Answer from the drawing. Dimensions are ordinates in mm from the lowest x, y and z of the part. A direction names the side the tool comes from. Round coordinates to 2 decimals unless told otherwise and drop trailing zeros. Loops run counter-clockwise (first coordinate to the right, second up) from the corner with the lowest first, then second, coordinate; pieces in that order, holes last.
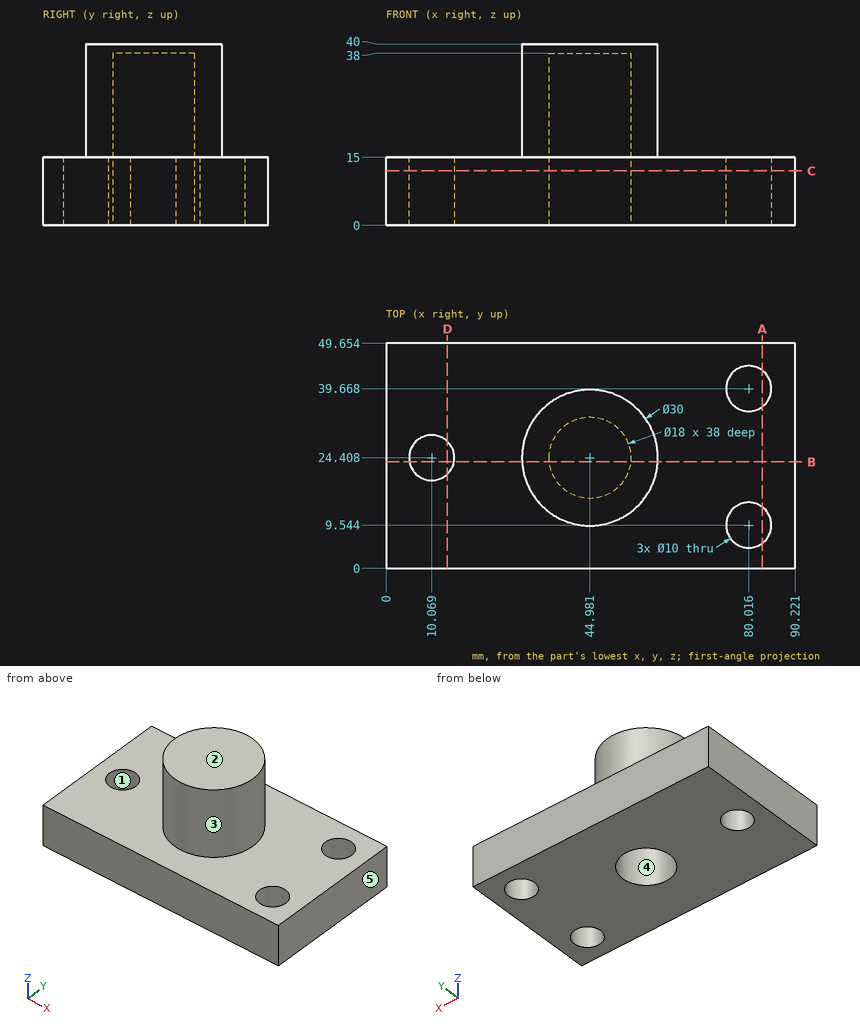
1. Find section B-B (y = 23.5). Write down the section's boundary in (x, z) (1 decimal).
Answer key:
outline: (0, 0) - (5.2, 0) - (5.2, 15) - (0, 15) - close; (15, 0) - (36, 0) - (36, 38) - (53.9, 38) - (53.9, 0) - (90.2, 0) - (90.2, 15) - (60, 15) - (60, 40) - (30, 40) - (30, 15) - (15, 15) - close
2. Find section A-A (x = 83). Write down the section's boundary in (y, z) (1 decimal).
Answer key:
outline: (0, 0) - (5.5, 0) - (5.5, 15) - (0, 15) - close; (13.6, 0) - (35.7, 0) - (35.7, 15) - (13.6, 15) - close; (43.7, 0) - (49.7, 0) - (49.7, 15) - (43.7, 15) - close
3. Find section C-C (z = 12). Write down the section's boundary in (x, y) (1 decimal).
Answer key:
outline: (0, 0) - (90.2, 0) - (90.2, 49.7) - (0, 49.7) - close; hole circle Ø10 at (10.1, 24.4); hole circle Ø18 at (45, 24.4); hole circle Ø10 at (80, 9.5); hole circle Ø10 at (80, 39.7)
4. Consider probe 1 along Z at (x, y) = (58.5, 3.5); probe 2 along X at (y, z) = (40, 8.5) (1 decimal); probe 3 along Y at (x, z) = (43, 6) (1 decimal). Determine where each line is inside the solid, lowest interval first.
Answer key:
probe 1: z = 0 to 15
probe 2: x = 0 to 75, 85 to 90.2
probe 3: y = 0 to 15.6, 33.2 to 49.7
5. Given pin 1 (4 mm diameter, centred on y = 27, z = 33, fed in from +X); pin 2 (6 mm diameter, centred on x = 51, z = 22.5, fed in from -Y) (1 decimal); pin 3 (4 mm diameter, centred on x = 11.5, y = 13.5, fed in from +Z), each flat-ended and moving along its own axis, determine where each tip first touches the part or whether it passes through.
Answer key:
pin 1: stops at x = 59.97
pin 2: stops at y = 9.7
pin 3: stops at z = 15
6. Determine the mould class of the marked faces 1, 2 and 3 for opening direction Y: +Y half, -Y half, draft (parallel to the pull), parting line (faces both ways), or undercut.
Answer key:
face 1: undercut
face 2: draft
face 3: parting line
7. Find section D-D (x = 13.5). Write down the section's boundary in (y, z) (1 decimal), then the cut area to 3 significant figures.
Answer key:
outline: (0, 0) - (20.8, 0) - (20.8, 15) - (0, 15) - close; (28, 0) - (49.7, 0) - (49.7, 15) - (28, 15) - close
area: 636 mm2
8. Which of the six approach directions +Z, -Z, +X, -X, +Y, -Y give full straight-line access (tool end or side, diameter ignored) to the marked faces 4 and 5?
Answer key:
face 4: -Z
face 5: +Z, -Z, +X, +Y, -Y
